Input: part model. Units: mm. Frame: model coordinates. Face numbers are marked on the shaded views. A direction names the side the tool comes from. Give positions to 0.01 mm unless a question says otherwise; leave off trailing zeros. Loops run counter-clockwise (first coordinate to the right, second up) from the corner with the lowest first, then second, coordinate; pieces in that order, holes last. Notation, with made-up numbers: M -11.75,38.25 L 9.25,38.25 A26 cw 9.25,76.25 Z; hole C 43.25,24 d11. An arc over 180 degrees is marked long. Use a Markdown table: item, result. Add a question column.
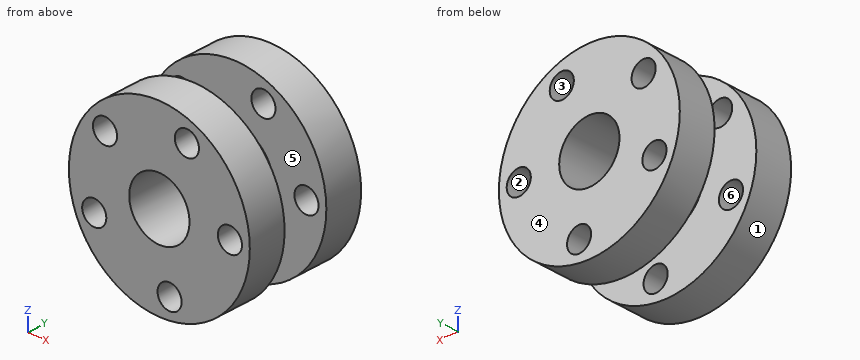
from build123d import *

# Parameters (mm, degrees)
F0_R     = 60
F1_DEPTH = 25
F2_R     = 25
F3_DEPTH = 30
F4_R     = 60
F5_DEPTH = 25
F6_R     = 20
F7_DEPTH = 80.001
F8_R     = 8
F9_DEPTH = 80.001


with BuildPart() as f1:
    # F0 (on Front) → F1 (new body)
    with BuildSketch(Plane.XZ):
        Circle(F0_R)
    extrude(amount=F1_DEPTH)

    # F2 (on face) → F3 (join)
    with BuildSketch(Plane(origin=(0, 0, 0), x_dir=(-1, 0, 0), z_dir=(0, 1, 0))):
        Circle(F2_R)
    extrude(amount=F3_DEPTH)

    # F4 (on face) → F5 (join)
    with BuildSketch(Plane(origin=(0, 30, 0), x_dir=(-1, 0, 0), z_dir=(0, 1, 0))):
        Circle(F4_R)
    extrude(amount=F5_DEPTH)

    # F6 (on face) → F7 (cut, through all)
    with BuildSketch(Plane.XZ.offset(25)):
        Circle(F6_R)
    extrude(amount=-F7_DEPTH, mode=Mode.SUBTRACT)

    # F8 (on face) → F9 (cut, through all)
    with BuildSketch(Plane.XZ.offset(25)):
        with Locations((-36.019197, 29.902987)):
            Circle(F8_R)
        with Locations((18.275928, 43.099439)):
            Circle(F8_R)
        with Locations((-43.162904, -18.125534)):
            Circle(F8_R)
        with Locations((46.81422, 0)):
            Circle(F8_R)
        with Locations((6.80161, -46.317484)):
            Circle(F8_R)
    extrude(amount=-F9_DEPTH, mode=Mode.SUBTRACT)


solid = f1.part
1) Ray query, line 1 (X direction, y = -10.5, z = 0.5); line 2 (Z direction, x = 16, y = 48); line 3 (Y direction, x = 28, z = 23.5). Return the intervals inside material, ascending. Write a range as [from, to].
2) Section query A-A, the plane z = 0. Return the cut outline in (x, y).
3) Section query C-C, the plane x = 43. Return the cut outline in (y, z), and give its area (3 significant figures).
4) Reachability of the marked faces 5 and 6 from +Z, -Z, +X, -X, +Y, -Y: full face, straight path, thin tool, end or side. Return the list, or none.
5) Contact query for flat-ended pins moving along their axis: P1, Ø4, axis at y = 30, z = -22, coming from the +X side; P2, Ø5, axis at x = 47.5, y = 4.5, coming from the -Z side; P3, Ø10, axis at x = -32.5, y = 37, coming from the -Z side; P4, Ø21, axis at x = -43.16, z = -18.13, coming from the -Y side. Output: stop coordinate, or through.
6) Section query B-B, the plane x = -14. Return the cut outline in (y, z).
7) Pull-direction query (Z, two-part tool) for the marked faces 1, 2, 3 and 4; classes: pulls with the +Z half, pulls with the -Z half, needs draft (parallel to the pull), parting line crosses it, or undercut.
8) Section query D-D, the plane y = 22.5. Return the cut outline in (x, z).
Entries:
| question | item | result |
|---|---|---|
| 1 | line 1 | x = [-60, -19.99], [19.99, 38.83], [54.8, 60] |
| 1 | line 2 | z = [-57.83, -12], [12, 35.43], [50.77, 57.83] |
| 1 | line 3 | y = [-25, 0], [30, 55] |
| 2 | outline | M -60,-25 L -20,-25 L -20,55 L -60,55 L -60,30 L -25,30 L -25,0 L -60,0 Z; M 20,-25 L 38.81,-25 L 38.81,0 L 25,0 L 25,30 L 38.81,30 L 38.81,55 L 20,55 Z; M 54.81,-25 L 60,-25 L 60,0 L 54.81,0 Z; M 54.81,30 L 60,30 L 60,55 L 54.81,55 Z |
| 3 | outline | M -25,-41.84 L 0,-41.84 L 0,-7.03 L -25,-7.03 Z; M -25,7.03 L 0,7.03 L 0,41.84 L -25,41.84 Z; M 30,-41.84 L 55,-41.84 L 55,-7.03 L 30,-7.03 Z; M 30,7.03 L 55,7.03 L 55,41.84 L 30,41.84 Z |
| 3 | area | 3,480 mm² |
| 4 | face 5 | none |
| 4 | face 6 | +Y, -Y |
| 5 | P1 | stops at x = 56.57 |
| 5 | P2 | passes through |
| 5 | P3 | stops at z = -53.33 |
| 5 | P4 | stops at y = -25 |
| 6 | outline | M -25,-58.34 L 0,-58.34 L 0,-20.71 L 30,-20.71 L 30,-58.34 L 55,-58.34 L 55,-14.28 L -25,-14.28 Z; M -25,14.28 L 55,14.28 L 55,58.34 L 30,58.34 L 30,20.71 L 0,20.71 L 0,58.34 L -25,58.34 Z |
| 7 | face 1 | parting line crosses it |
| 7 | face 2 | undercut |
| 7 | face 3 | undercut |
| 7 | face 4 | needs draft |
| 8 | outline | C 0,0 d50; hole C 0,0 d40 |
